Autodesk Inventor part; units mm, degrees
ref_plane "YZ Plane" through (0, 0, 0) normal (1, 0, 0) x (0, 1, 0)
ref_plane "XZ Plane" through (0, 0, 0) normal (0, 1, 0) x (-1, 0, 0)
ref_plane "XY Plane" through (0, 0, 0) normal (0, 0, 1) x (1, 0, 0)
sketch "Sketch1" plane through (0, 0, 0) normal (0, 1, 0) x (-1, 0, 0)
  line L0 (0, 0) -> (381, 0)
  line L1 (381, 0) -> (381, -1524)
  line L2 (381, -1524) -> (0, -1524)
  line L3 (0, -1524) -> (0, 0)
  dimension "d0" = 381
  dimension "d1" = 1524
extrude "Extrusion1" add sketch "Sketch1" along normal blind 635
fillet "Fillet1" radius 203.2 1 edges at (-381, 635, -762)
sketch "Sketch2" plane through (0, 0, 0) normal (1, 0, 0) x (0, 0, -1)
  line L0 (101.6, 44.45) -> (355.6, 44.45)
  line L1 (355.6, 44.45) -> (355.6, 298.45)
  line L2 (355.6, 298.45) -> (101.6, 298.45)
  line L3 (101.6, 298.45) -> (101.6, 44.45)
  line L4 (0, 0) -> (1524, 0)
  line L5 (101.6, 590.55) -> (355.6, 590.55)
  line L6 (355.6, 590.55) -> (355.6, 336.55)
  line L7 (355.6, 336.55) -> (101.6, 336.55)
  line L8 (101.6, 336.55) -> (101.6, 590.55)
  line L9 (0, 0) -> (0, 635)
  line L10 (457.2, 590.55) -> (711.2, 590.55)
  line L11 (711.2, 590.55) -> (711.2, 336.55)
  line L12 (711.2, 336.55) -> (457.2, 336.55)
  line L13 (457.2, 336.55) -> (457.2, 590.55)
  line L14 (457.2, 298.45) -> (711.2, 298.45)
  line L15 (711.2, 298.45) -> (711.2, 44.45)
  line L16 (711.2, 44.45) -> (457.2, 44.45)
  line L17 (457.2, 44.45) -> (457.2, 298.45)
  line L18 (812.8, 590.55) -> (1066.8, 590.55)
  line L19 (1066.8, 590.55) -> (1066.8, 336.55)
  line L20 (1066.8, 336.55) -> (812.8, 336.55)
  line L21 (812.8, 336.55) -> (812.8, 590.55)
  line L22 (812.8, 298.45) -> (1066.8, 298.45)
  line L23 (1066.8, 298.45) -> (1066.8, 44.45)
  line L24 (1066.8, 44.45) -> (812.8, 44.45)
  line L25 (812.8, 44.45) -> (812.8, 298.45)
  line L26 (1168.4, 590.55) -> (1422.4, 590.55)
  line L27 (1422.4, 590.55) -> (1422.4, 336.55)
  line L28 (1422.4, 336.55) -> (1168.4, 336.55)
  line L29 (1168.4, 336.55) -> (1168.4, 590.55)
  line L30 (1168.4, 286.2198) -> (1422.4, 286.2198)
  line L31 (1422.4, 286.2198) -> (1422.4, 32.2198)
  line L32 (1422.4, 32.2198) -> (1168.4, 32.2198)
  line L33 (1168.4, 32.2198) -> (1168.4, 286.2198)
  dimension "d5" = 254
  dimension "d6" = 254
  dimension "d7" = 44.45
  dimension "d8" = 254
  dimension "d9" = 38.1
  dimension "d10" = 101.6
  dimension "d11" = 254
  dimension "d12" = 101.6
  dimension "d13" = 254
  dimension "d14" = 254
  dimension "d15" = 101.6
  dimension "d16" = 101.6
  dimension "d17" = 254
  dimension "d18" = 101.6
  dimension "d19" = 254
  dimension "d20" = 101.6
  dimension "d21" = 254
  dimension "d22" = 254
extrude "Extrusion2" cut sketch "Sketch2" against normal blind 76.2
sketch "Sketch3" plane through (-76.2, 0, 0) normal (1, 0, 0) x (0, 0, -1)
  line L0 (101.6, 336.55) -> (101.6, 590.55)
  line L1 (355.6, 336.55) -> (101.6, 336.55)
  line L2 (101.6, 590.55) -> (355.6, 590.55)
  line L3 (355.6, 590.55) -> (355.6, 336.55)
  line L4 (355.6, 336.55) -> (101.6, 336.55)
  line L5 (101.6, 336.55) -> (101.6, 590.55)
  circle A0 centre (228.6, 463.55) radius 101.6
  point P0 (0, 0)
  dimension "d25" = 127
  dimension "d26" = 127
  dimension "d27" = 203.2
sketch "Sketch5" plane through (-76.2, 0, 0) normal (1, 0, 0) x (0, 0, -1)
  line L0 (101.6, 298.45) -> (355.6, 298.45)
  line L1 (101.6, 298.45) -> (355.6, 298.45)
  line L2 (355.6, 298.45) -> (355.6, 44.45)
  line L3 (355.6, 44.45) -> (101.6, 44.45)
  line L4 (101.6, 44.45) -> (101.6, 298.45)
  circle A0 centre (228.6, 171.45) radius 101.6
  point P0 (0, 0)
  dimension "d28" = 203.2
sketch "Sketch6" plane through (-76.2, 0, 0) normal (1, 0, 0) x (0, 0, -1)
  line L0 (457.2, 336.55) -> (457.2, 590.55)
  line L1 (457.2, 590.55) -> (711.2, 590.55)
  line L2 (711.2, 590.55) -> (711.2, 336.55)
  line L3 (711.2, 336.55) -> (457.2, 336.55)
  line L4 (457.2, 336.55) -> (457.2, 590.55)
  circle A0 centre (584.2, 463.55) radius 101.6
  point P0 (0, 0)
  dimension "d29" = 203.2
sketch "Sketch7" plane through (-76.2, 0, 0) normal (1, 0, 0) x (0, 0, -1)
  line L0 (711.2, 44.45) -> (457.2, 44.45)
  line L1 (457.2, 44.45) -> (711.2, 44.45)
  line L2 (711.2, 44.45) -> (711.2, 298.45)
  line L3 (711.2, 298.45) -> (457.2, 298.45)
  line L4 (457.2, 298.45) -> (457.2, 44.45)
  circle A0 centre (584.2, 171.45) radius 101.6
  point P0 (0, 0)
  dimension "d30" = 203.2
sketch "Sketch8" plane through (-76.2, 0, 0) normal (1, 0, 0) x (0, 0, -1)
  line L0 (812.8, 336.55) -> (812.8, 590.55)
  line L1 (1066.8, 590.55) -> (1066.8, 336.55)
  line L2 (812.8, 590.55) -> (1066.8, 590.55)
  line L3 (1066.8, 590.55) -> (1066.8, 336.55)
  line L4 (1066.8, 336.55) -> (812.8, 336.55)
  line L5 (812.8, 336.55) -> (812.8, 590.55)
  circle A0 centre (939.8, 463.55) radius 101.6
  point P0 (0, 0)
  dimension "d31" = 203.2
sketch "Sketch9" plane through (-76.2, 0, 0) normal (1, 0, 0) x (0, 0, -1)
  line L0 (812.8, 298.45) -> (1066.8, 298.45)
  line L1 (1066.8, 298.45) -> (1066.8, 44.45)
  line L2 (1066.8, 44.45) -> (812.8, 44.45)
  line L3 (812.8, 44.45) -> (812.8, 298.45)
  circle A0 centre (939.8, 171.45) radius 101.6
  point P0 (0, 0)
  dimension "d32" = 203.2
sketch "Sketch10" plane through (-76.2, 0, 0) normal (1, 0, 0) x (0, 0, -1)
  line L0 (1168.4, 336.55) -> (1168.4, 590.55)
  line L1 (1422.4, 590.55) -> (1422.4, 336.55)
  line L2 (1168.4, 590.55) -> (1422.4, 590.55)
  line L3 (1422.4, 590.55) -> (1422.4, 336.55)
  line L4 (1422.4, 336.55) -> (1168.4, 336.55)
  line L5 (1168.4, 336.55) -> (1168.4, 590.55)
  circle A0 centre (1295.4, 463.55) radius 101.6
  point P0 (0, 0)
  dimension "d33" = 203.2
sketch "Sketch11" plane through (-76.2, 0, 0) normal (1, 0, 0) x (0, 0, -1)
  line L0 (1422.4, 286.2198) -> (1422.4, 32.2198)
  line L1 (1168.4, 286.2198) -> (1422.4, 286.2198)
  line L2 (1422.4, 286.2198) -> (1422.4, 32.2198)
  line L3 (1422.4, 32.2198) -> (1168.4, 32.2198)
  line L4 (1168.4, 32.2198) -> (1168.4, 286.2198)
  circle A0 centre (1295.4, 159.2198) radius 101.6
  point P0 (0, 0)
  dimension "d34" = 203.2
extrude "Extrusion3" add sketch "Sketch3" along normal blind 50.8 contours A0
extrude "Extrusion4" add sketch "Sketch6" along normal blind 50.8 contours A0
extrude "Extrusion5" add sketch "Sketch8" along normal blind 50.8 contours A0
extrude "Extrusion6" add sketch "Sketch10" along normal blind 50.8 contours A0
extrude "Extrusion7" add sketch "Sketch5" along normal blind 50.8 contours A0
extrude "Extrusion8" add sketch "Sketch7" along normal blind 50.8 contours A0
extrude "Extrusion9" add sketch "Sketch9" along normal blind 50.8 contours A0
extrude "Extrusion10" add sketch "Sketch11" along normal blind 50.8 contours A0
sketch "Sketch12" plane through (0, 635, 0) normal (0, 1, 0) x (1, 0, 0)
  circle A0 centre (-88.9, 635) radius 63.5
  line L0 (0, 0) -> (0, 1524)
  line L1 (-177.8, 0) -> (0, 0)
  circle A1 centre (-88.9, 889) radius 63.5
  line L2 (0, 1524) -> (-177.8, 1524)
  dimension "d51" = 127
  dimension "d52" = 88.9
  dimension "d53" = 635
  dimension "d54" = 127
  dimension "d55" = 88.9
  dimension "d56" = 635
extrude "Extrusion11" add sketch "Sketch12" along normal blind 127
fillet "Fillet2" radius 25.4 2 edges at (0, 317.5, 0) (-152.4, 762, -635)
fillet "Fillet3" radius 25.4 1 edges at (-152.4, 762, -889)
fillet "Fillet4" radius 25.4 1 edges at (0, 317.5, -1524)
properties part number "PTreasureChestFinal-ver1-1111-2021"
CAD build for the part. Positions are in the model's coordinates, mm. A direction names the side the tool comes from. Round coordinates to 2 decimals unless told otherwise and drop trailing zeros. Loops run counter-clockwise (first coordinate to the right, second up) from the corner with the lowest first, then second, coordinate; pieces in that order, holes last.
(1) Cut at A-A (y = 701). Give the cut face in (x, z), plus the area to 3 significant figures.
(2) Cut at C-C (x = -218). Give the cut face in (y, z).
(3) Wall check: line 1 along Y through (x, z) = (-23.5, -907.5); line 2 along Y through (x, z) = (-40, -1273); line 3 along X through (y, z) = (282.5, -931). Give the ranges that are in metal, low to high.
(4) Two-plate mould, pull along Z, no slides. Class faces 1 (the flat face through (-38, 462, -1168.4)), 2 (the flat face through (-89, 762, -890)): +Z half, -Z half, draft (parallel to the pull), parting line (faces both ways), or undercut.
(5) Cut at B-B (z = -394). Give the cut face in (x, y), plus the area to 3 significant figures.
(6) Which spindle directions (+Z, -Z, +X, -X, +Y, -Y) get a long thin tool onto all of the face, cutting with end or side? Do faces 3 (the flat face through (-25.4, 465, -583)), 4 (the cylindrical face through (-102.67, 685.09, -696.99)), 5 (the flat face through (-89, 762, -636)). Say none if no direction does.
(7) Drop flat-ended pins along their axis: pin 1 (4 mm diameter, centred on x = -271, z = -658, fed in from +Y); pin 2 (1 mm diameter, centred on x = -283, z = -1129, fed in from +Y); pin 3 (1.5 mm diameter, centred on x = -175, z = -1153.5, fed in from +Y). Give the stop position or say it passes through.
(8) Cut at D-D (z = -228.6). Give the cut face in (x, y), plus the area to 3 significant figures.
Findings below:
1. outline: circle Ø127 at (-88.9, -889); circle Ø127 at (-88.9, -635)
1. area: 25,300 mm2
2. outline: (0, -1524) - (630.98, -1524) - (630.98, 0) - (0, 0) - close
3. line 1: y = 0 to 44.45, 298.45 to 336.55, 590.55 to 635
3. line 2: y = 0 to 32.22, 60.12 to 258.32, 286.22 to 336.55, 364.45 to 562.65, 590.55 to 635
3. line 3: x = -381 to -76.2
4. face 1: undercut
4. face 2: draft
5. outline: (-381, 0) - (0, 0) - (0, 635) - (-177.8, 635) arc R203.2 ccw to (-381, 431.8) - close
5. area: 233,000 mm2
6. face 3: +X
6. face 4: +Y
6. face 5: +Z, -Z, +X, -X, +Y
7. pin 1: stops at y = 613.38
7. pin 2: stops at y = 605.95
7. pin 3: stops at y = 635
8. outline: (-381, 0) - (0, 0) - (0, 44.45) - (-76.2, 44.45) - (-76.2, 69.85) - (-25.4, 69.85) - (-25.4, 273.05) - (-76.2, 273.05) - (-76.2, 298.45) - (0, 298.45) - (0, 336.55) - (-76.2, 336.55) - (-76.2, 361.95) - (-25.4, 361.95) - (-25.4, 565.15) - (-76.2, 565.15) - (-76.2, 590.55) - (0, 590.55) - (0, 635) - (-177.8, 635) arc R203.2 ccw to (-381, 431.8) - close
8. area: 215,000 mm2
